from build123d import *

# Parameters (mm, degrees)
SKETCH_1_W               = 60
SKETCH_1_H               = 80
EXTRUDE_1_DEPTH          = 10
SKETCH_2_W               = 60
SKETCH_2_H               = 10
EXTRUDE_2_DEPTH          = 50
SKETCH_3_W               = 60
SKETCH_3_H               = 10
EXTRUDE_3_DEPTH          = 50
SKETCH_4_W               = 40
SKETCH_4_H               = 20
EXTRUDE_4_DEPTH          = 10
SKETCH_5_W               = 40
SKETCH_5_H               = 20
EXTRUDE_5_DEPTH          = 30
SKETCH_6_W               = 20
SKETCH_6_H               = 20
CUT_EXTRUDE_1_DEPTH      = 50
FILLET_1_R               = 10
CUT_EXTRUDE_2_DEPTH      = 50
CUT_EXTRUDE_2_DEPTH_BACK = 50
SKETCH_7_R               = 10


with BuildPart() as part:
    # 스케치1 → 보스-돌출1 (new body)
    with BuildSketch(Plane(origin=(0, 0, 0), x_dir=(1, 0, 0), z_dir=(0, 1, 0))):
        with Locations((30, 40)):
            Rectangle(SKETCH_1_W, SKETCH_1_H)
    extrude(amount=EXTRUDE_1_DEPTH)

    # 스케치2 → 보스-돌출2 (add)
    with BuildSketch(Plane(origin=(0, 10, 0), x_dir=(1, 0, 0), z_dir=(0, 1, 0))):
        with Locations((30, 75)):
            Rectangle(SKETCH_2_W, SKETCH_2_H)
    extrude(amount=EXTRUDE_2_DEPTH)

    # 스케치3 → 보스-돌출3 (add)
    with BuildSketch(Plane.XY.offset(-70)):
        with Locations((30, 35)):
            Rectangle(SKETCH_3_W, SKETCH_3_H)
    extrude(amount=EXTRUDE_3_DEPTH)

    # 스케치4 → 보스-돌출4 (add)
    with BuildSketch(Plane.XY.offset(-70)):
        with Locations((30, 20)):
            Rectangle(SKETCH_4_W, SKETCH_4_H)
    extrude(amount=EXTRUDE_4_DEPTH)

    # 스케치5 → 보스-돌출5 (add)
    with BuildSketch(Plane.XY.offset(-70)):
        with Locations((30, 50)):
            Rectangle(SKETCH_5_W, SKETCH_5_H)
    extrude(amount=EXTRUDE_5_DEPTH)

    # 스케치6 → 컷-돌출1 (cut)
    with BuildSketch(Plane.XY.offset(-40)):
        with Locations((30, 50)):
            Rectangle(SKETCH_6_W, SKETCH_6_H)
    extrude(amount=-CUT_EXTRUDE_1_DEPTH, mode=Mode.SUBTRACT)

    # 필렛1
    fillet_1_edges = [part.edges().sort_by_distance(p)[0] for p in [
        (0, 60, -75),
        (60, 60, -75),
        (0, 35, -20),
        (60, 35, -20),
        (60, 5, 0),
        (0, 5, 0),
    ]]
    fillet(fillet_1_edges, radius=FILLET_1_R)

    # 스케치7 → 컷-돌출2 (cut, two sides: drawn at the far end of the back side and taken through both)
    with BuildSketch(Plane(origin=(0, 10, 0), x_dir=(1, 0, 0), z_dir=(0, 1, 0)).offset(-CUT_EXTRUDE_2_DEPTH_BACK)):
        with Locations(Location((30, 40, 0), (0, 0, 90))):
            Circle(SKETCH_7_R)
    extrude(amount=CUT_EXTRUDE_2_DEPTH + CUT_EXTRUDE_2_DEPTH_BACK, mode=Mode.SUBTRACT)


solid = part.part
The model under review builds one solid part; all positions refer to its coordinate system, in mm. A direction names the side the tool comes from. Give positions to 0.01 mm unless a question says otherwise; leave off trailing zeros. Order: outer loops, then holes, each group sorted by start corner. A loop starts at its lowest first (then second) coordinate and runs counter-clockwise, first axis right, second up. Notation, with made-up numbers: (83, 70) -> (130, 70) arc R18 cw to (130, 90) -> close; hole circle Ø9 at (-31.5, 48.25). An arc over 180 degrees is marked (long way). Write item = value, one per line. Start each with the question number.
(1) Draft analysis for pull direction Z (two halves, no side actions). For faces 1 (the cylindrical face through (39.76, 34.93, -37.83)), 2 (the flat face through (30, 30, -80)), 3 (the flat face through (55, 20, -70)), 4 (the flat face through (10, 50, -55)), state which applies: +Z half, -Z half, draft (parallel to the pull), parting line (faces both ways), or undercut.
(2) Take a section at D-D (y = 5.5). Write out the cut boundary in (x, z).
(3) For L1, parallel to X at y = 2.75, z = -40; L2, parallel to Y at x = 13, z = -50.5; L3, parallel to Y at x = 58.5, z = -50, list the stretches that pass through material, from the lowest coordinate up. Write a range as from..to.
(4) Take a section at A-A (y = 43). Write out the cut boundary in (x, z).
(5) Tool access review of faces 5 (the flat face through (50, 50, -55)), 6 (the flat face through (45, 50, -40)), 7 (the flat face through (50, 20, -65)), 8 (the flat face through (30, 40, -65)), 9 (the flat face through (5, 20, -70)): name each direction out of +Z, -Z, +X, -X, +Y, -Y from which nothing blocks a thin tool from reaching the whole face with its end or side.
(6) Take a section at B-B (x = 22). Write out the cut boundary in (y, z).
(7) For pin 1 Ø3 at (x, y) = (3, 19.5) entering from +Z; pin 2 Ø8 at (y, z) = (24, -65) entering from -X; pin 3 Ø16 at (x, z) = (30, -40) entering from +Y; pin 4 Ø5 at (x, y) = (28, 37) entering from +Z, all flat-tipped, find the tip position at first contact; note any pin that passes through.
(8) Take a section at C-C (z = -67.5). Write out the cut boundary in (x, y), plus the area to 3 significant figures.
Returned:
q1.face_1 = undercut
q1.face_2 = -Z half
q1.face_3 = +Z half
q1.face_4 = draft
q2.outline = (0, -80) -> (60, -80) -> (60, -10) arc R10 ccw to (50, 0) -> (10, 0) arc R10 ccw to (0, -10) -> close; hole circle Ø20 at (30, -40)
q3.L1 = 0..20, 40..60
q3.L2 = 0..10, 30..60
q3.L3 = 0..10, 30..40
q4.outline = (0, -80) -> (20, -80) -> (20, -40) -> (10, -40) -> (10, -70) -> (0, -70) -> close; (40, -80) -> (60, -80) -> (60, -70) -> (50, -70) -> (50, -40) -> (40, -40) -> close
q5.face_5 = +Z, +X, +Y
q5.face_6 = +Z, +X, -X, +Y
q5.face_7 = +Z, +X
q5.face_8 = +Z, -Z, +Y
q5.face_9 = +Z, -X
q6.outline = (0, -80) -> (40, -80) -> (40, -46) -> (30, -46) -> (30, -60) -> (10, -60) -> (10, -46) -> (0, -46) -> close; (0, -34) -> (10, -34) -> (10, 0) -> (0, 0) -> close; (30, -34) -> (40, -34) -> (40, -20) -> (30, -20) -> close
q7.pin_1 = -70
q7.pin_2 = 10
q7.pin_3 = through
q7.pin_4 = -20
q8.outline = (0, 0) -> (60, 0) -> (60, 10) -> (50, 10) -> (50, 30) -> (60, 30) -> (60, 40) -> (50, 40) -> (50, 60) -> (40, 60) -> (40, 40) -> (20, 40) -> (20, 60) -> (10, 60) -> (10, 40) -> (0, 40) -> (0, 30) -> (10, 30) -> (10, 10) -> (0, 10) -> close
q8.area = 2,400 mm²
